Can you work these out from the model? Positions are in its coordinate system, mm. A direction names the side the tool comes from. Round coordinates to 2 decimals unless told otherwise and drop trailing zeros. Loops run counter-clockwise (first coordinate to the right, second up) from the corner with the lowest first, then second, coordinate; pieces in that order, holes last. Notation, with made-up numbers: M 39.25,-2.5 L 83.25,-2.5 A27 ccw 83.25,36.5 Z; hole C 10.25,-28.5 d7. An arc over 180 degrees is marked long. Answer as CSV lines item,"result".
from build123d import *

# Parameters (mm, degrees)
SKETCH1_W           = 800
SKETCH1_H           = 1200
BOSS_EXTRUDE1_DEPTH = 500
SKETCH2_W           = 700
SKETCH2_H           = 320
CUT_EXTRUDE1_DEPTH  = 400


with BuildPart() as part:
    # Sketch1 → Boss-Extrude1 (new body)
    with BuildSketch(Plane.XY):
        Rectangle(SKETCH1_W, SKETCH1_H)
    extrude(amount=BOSS_EXTRUDE1_DEPTH)

    # Sketch2 → Cut-Extrude1 (cut)
    with BuildSketch(Plane.XY.offset(500)):
        with Locations((0, 380)):
            Rectangle(SKETCH2_W, SKETCH2_H)
        Rectangle(SKETCH2_W, SKETCH2_H)
        with Locations((0, -380)):
            Rectangle(SKETCH2_W, SKETCH2_H)
    extrude(amount=-CUT_EXTRUDE1_DEPTH, mode=Mode.SUBTRACT)


solid = part.part
Item 1: We'd pull the mould along Y, two halves only. Please class faces 3 (the face through (-5, -378, 100)), 4 (the face through (400, -8, 246)), 5 (the face through (-6, 600, 246)): released by +Y, released by -Y, zero draft, split by the parting line, or undercut.
Output:
face 3,"undercut"
face 4,"zero draft"
face 5,"released by +Y"
Item 2: If we section it at A-A on y = -51.5: Write out the boundary of the cut face in (x, z).
Output:
outline,"M -400,0 L 400,0 L 400,500 L 350,500 L 350,100 L -350,100 L -350,500 L -400,500 Z"
Item 3: On a 3-axis mill with a long thin cutter (end or side, diameter ignored), from which of +Z, -Z, +X, -X, +Y, -Y can I reach the whole of each face in a straight line? I mean faces 1 (the face through (350, -2, 303)), 2 (the face through (-6, 8, 0)). Say none if no direction works.
Output:
face 1,"+Z"
face 2,"-Z, +X, -X, +Y, -Y"
Item 4: If I drill on line 1 along Y through (x, z) = (-231, 424.5); line 2 along X through (y, z) = (-376.5, 230.5); line 3 along Z through (x, y) = (-184.5, 484), over which ranges is the centre line in solid material (lowest first)? Write a range as from..to.
Output:
line 1,"y = -600..-540, -220..-160, 160..220, 540..600"
line 2,"x = -400..-350, 350..400"
line 3,"z = 0..100"
Item 5: If we section it at B-B on z = 222: Write out the boundary of the cut face in (x, y), then the cut area to 3 significant figures.
Output:
outline,"M -400,-600 L 400,-600 L 400,600 L -400,600 Z; hole M -350,-540 L 350,-540 L 350,-220 L -350,-220 Z; hole M -350,-160 L 350,-160 L 350,160 L -350,160 Z; hole M -350,220 L 350,220 L 350,540 L -350,540 Z"
area,"288,000 mm2"
Item 6: Will these pins go through, and if not, where does the flat tip stop? pin 1 (10 mm diameter, centred on x = 209, y = 102.5, fed in from -Z); pin 2 (2 mm diameter, centred on x = -190.5, y = 369.5, fed in from +Z).
Output:
pin 1,"stops at z = 0"
pin 2,"stops at z = 100"
Item 7: If we section it at C-C on x = 259: Write out the boundary of the cut face in (y, z), then the cut area to 3 significant figures.
Output:
outline,"M -600,0 L 600,0 L 600,500 L 540,500 L 540,100 L 220,100 L 220,500 L 160,500 L 160,100 L -160,100 L -160,500 L -220,500 L -220,100 L -540,100 L -540,500 L -600,500 Z"
area,"216,000 mm2"
